Part model, mm, in its own coordinate system. Round coordinates to 2 decimals unless told otherwise and drop trailing zeros. Order: outer loops, then holes, each group sorted by start corner. A loop starts at its lowest first (then second) coordinate and runs counter-clockwise, first axis right, second up. Notation, with made-up numbers: M 75,43.25 L 98,43.25 A22 ccw 98,55.25 Z; hole C 47.5,61 d2. An arc over 180 degrees is marked long. Write each question's results on one line, items separated by ' | '. Start each with the question number.
1. Band-saw the part on D-D, the plane z = -85. List the corners of the cut face in (x, y) (3 decimals), then the cut area to 3 significant figures.
2. Band-saw the part on A-A, the plane y = 0. List the corners of the cut face in (x, z) (3 decimals), then the cut area to 3 significant figures.
3. Band-saw the part on C-C, the plane z = -127. List the corners of the cut face in (x, y) (3 decimals), then the cut area to 3 significant figures.
4. Probe L1, parallel to Z at x = -2.25, y = -23; L2, parallel to Z at x = -6, y = 8.5; L3, parallel to X at y = 3.5, z = -57.5 (3 decimals). List the from-to ranges inside material, lowest first. Write a range as [from, to].
5. Band-saw the part on B-B, the plane x = -7. Give the number of separate pieces and of enclosed holes in the cut face, then the cut area to 3 significant figures.
6. Drop flat-ended pins along their axis: pin 1 Ø8 at (y, z) = (-7.76, -28.98) entering from -X; pin 2 Ø2 at (x, z) = (-6.5, -50.5) entering from -Y; pin 3 Ø1.7 at (x, y) = (-4, -24) entering from +Z. Give the stop position or say it passes through.
```python
from build123d import *

# Parameters (mm, degrees)
SKETCH1_R           = 35
SKETCH1_R_2         = 22.5
SKETCH1_R_3         = 2.25
BOSS_EXTRUDE1_DEPTH = 2.5
SKETCH2_R           = 22.5
SKETCH2_R_2         = 2.25
SKETCH2_R_3         = 3.2639
BOSS_EXTRUDE2_DEPTH = 7.025
CUT_EXTRUDE1_DEPTH  = 146.433749952
SKETCH4_R           = 5
CUT_EXTRUDE2_DEPTH  = 4.525


with BuildPart() as part:
    # Sketch1 → Boss-Extrude1 (new body)
    with BuildSketch(Plane.ZY):
        Circle(SKETCH1_R)
        Circle(SKETCH1_R_2, mode=Mode.SUBTRACT)
        with Locations((-21.213203436, -21.213203436)):
            Circle(SKETCH1_R_3, mode=Mode.SUBTRACT)
        with Locations((-28.977774789, -7.764571353)):
            Circle(SKETCH1_R_3, mode=Mode.SUBTRACT)
        with Locations((-28.977774789, 7.764571353)):
            Circle(SKETCH1_R_3, mode=Mode.SUBTRACT)
        with Locations((-21.213203436, 21.213203436)):
            Circle(SKETCH1_R_3, mode=Mode.SUBTRACT)
        with Locations((-7.764571353, 28.977774789)):
            Circle(SKETCH1_R_3, mode=Mode.SUBTRACT)
        with Locations((7.764571353, 28.977774789)):
            Circle(SKETCH1_R_3, mode=Mode.SUBTRACT)
        with Locations((21.213203436, 21.213203436)):
            Circle(SKETCH1_R_3, mode=Mode.SUBTRACT)
        with Locations((28.977774789, 7.764571353)):
            Circle(SKETCH1_R_3, mode=Mode.SUBTRACT)
        with Locations((28.977774789, -7.764571353)):
            Circle(SKETCH1_R_3, mode=Mode.SUBTRACT)
        with Locations((21.213203436, -21.213203436)):
            Circle(SKETCH1_R_3, mode=Mode.SUBTRACT)
    extrude(amount=BOSS_EXTRUDE1_DEPTH)

    # Sketch2 → Boss-Extrude2 (add)
    with BuildSketch(Plane.ZY.offset(2.5)):
        with BuildLine():
            Line((0, 40), (-30, 40))
            ThreePointArc((-30, 40), (-37.274117863, 39.468042303), (-44.393454807, 37.883488373))
            Line((-44.393454807, 37.883488373), (-130.598363702, 11.970872093))
            ThreePointArc((-130.598363702, 11.970872093), (-139.5, 0), (-130.598363702, -11.970872093))
            Line((-130.598363702, -11.970872093), (-44.393454807, -37.883488373))
            ThreePointArc((-44.393454807, -37.883488373), (-37.274117863, -39.468042303), (-30, -40))
            Line((-30, -40), (0, -40))
            ThreePointArc((0, -40), (40, 0), (0, 40))
        make_face()
        Circle(SKETCH2_R, mode=Mode.SUBTRACT)
        with Locations((-21.213203436, -21.213203436)):
            Circle(SKETCH2_R_2, mode=Mode.SUBTRACT)
        with Locations((-28.977774789, -7.764571353)):
            Circle(SKETCH2_R_2, mode=Mode.SUBTRACT)
        with Locations((-28.977774789, 7.764571353)):
            Circle(SKETCH2_R_2, mode=Mode.SUBTRACT)
        with Locations((-21.213203436, 21.213203436)):
            Circle(SKETCH2_R_2, mode=Mode.SUBTRACT)
        with Locations((-7.764571353, 28.977774789)):
            Circle(SKETCH2_R_2, mode=Mode.SUBTRACT)
        with Locations((7.764571353, 28.977774789)):
            Circle(SKETCH2_R_2, mode=Mode.SUBTRACT)
        with Locations((21.213203436, 21.213203436)):
            Circle(SKETCH2_R_2, mode=Mode.SUBTRACT)
        with Locations((28.977774789, 7.764571353)):
            Circle(SKETCH2_R_2, mode=Mode.SUBTRACT)
        with Locations((28.977774789, -7.764571353)):
            Circle(SKETCH2_R_2, mode=Mode.SUBTRACT)
        with Locations((21.213203436, -21.213203436)):
            Circle(SKETCH2_R_2, mode=Mode.SUBTRACT)
        with Locations((-127, 0)):
            Circle(SKETCH2_R_3, mode=Mode.SUBTRACT)
    extrude(amount=BOSS_EXTRUDE2_DEPTH)

    # Sketch3 → Cut-Extrude1 (cut, through all)
    with BuildSketch(Plane(origin=(0, 0, 0), x_dir=(0, 0, -1), z_dir=(1, 0, 0))):
        with BuildLine():
            Line((26.998480774, -40), (0, -40))
            ThreePointArc((0, -40), (-12.729354805, -37.920489531), (-24.135168281, -31.898176312))
            ThreePointArc((-24.135168281, -31.898176312), (-17.31861983, -32.534635526), (-13.713203436, -26.714722661))
            Line((-13.713203436, -26.714722661), (-13.713203436, -21.213203436))
            ThreePointArc((-13.713203436, -21.213203436), (-14.284106942, -18.343077693), (-15.909902577, -15.909902577))
            ThreePointArc((-15.909902577, -15.909902577), (0, -22.5), (15.909902577, -15.909902577))
            ThreePointArc((15.909902577, -15.909902577), (14.284106942, -18.343077693), (13.713203436, -21.213203436))
            Line((13.713203436, -21.213203436), (13.713203436, -26.714722661))
            ThreePointArc((13.713203436, -26.714722661), (17.604371078, -36.108832357), (26.998480774, -40))
        make_face()
    extrude(amount=-CUT_EXTRUDE1_DEPTH, mode=Mode.SUBTRACT)

    # Sketch4 → Cut-Extrude2 (cut)
    with BuildSketch(Plane.ZY.offset(9.525)):
        with Locations((-21.213203436, -21.213203436)):
            Circle(SKETCH4_R)
        with Locations((-28.977774789, -7.764571353)):
            Circle(SKETCH4_R)
        with Locations((-28.977774789, 7.764571353)):
            Circle(SKETCH4_R)
        with Locations((-21.213203436, 21.213203436)):
            Circle(SKETCH4_R)
        with Locations((-7.764571353, 28.977774789)):
            Circle(SKETCH4_R)
        with Locations((7.764571353, 28.977774789)):
            Circle(SKETCH4_R)
        with Locations((21.213203436, 21.213203436)):
            Circle(SKETCH4_R)
        with Locations((28.977774789, 7.764571353)):
            Circle(SKETCH4_R)
        with Locations((28.977774789, -7.764571353)):
            Circle(SKETCH4_R)
        with Locations((21.213203436, -21.213203436)):
            Circle(SKETCH4_R)
    extrude(amount=-CUT_EXTRUDE2_DEPTH, mode=Mode.SUBTRACT)


solid = part.part
```
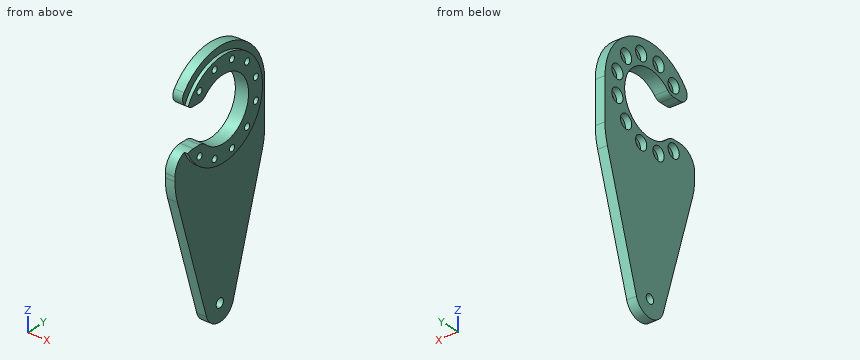
Solution:
1) outline: M -9.525,-25.677 L -2.5,-25.677 L -2.5,25.677 L -9.525,25.677 Z | area: 361 mm^2
2) outline: M -9.525,-139.5 L -2.5,-139.5 L -2.5,-130.264 L -9.525,-130.264 Z; M -9.525,-123.736 L -2.5,-123.736 L -2.5,-35 L 0,-35 L 0,-22.5 L -9.525,-22.5 Z; M -9.525,22.5 L 0,22.5 L 0,35 L -2.5,35 L -2.5,40 L -9.525,40 Z | area: 962 mm^2
3) outline: M -9.525,-13.053 L -2.5,-13.053 L -2.5,-3.264 L -9.525,-3.264 Z; M -9.525,3.264 L -2.5,3.264 L -2.5,13.053 L -9.525,13.053 Z | area: 138 mm^2
4) L1: [-26.38, -22.58], [-19.85, -13.71], [13.71, 19.85], [22.58, 26.38] | L2: [-136.17, -33.92], [-24.03, -20.83], [20.83, 24.03], [33.92, 39.09] | L3: [-9.525, -2.5]
5) separate pieces: 1 | enclosed holes: 11 | area: 7,510 mm^2
6) pin 1: x = -5 | pin 2: y = -36.35 | pin 3: z = 32.62
